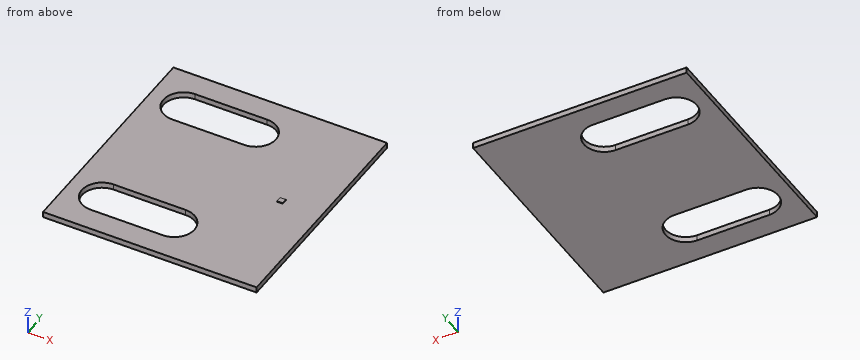
from build123d import *

# Parameters (mm, degrees)
SKETCH1_W           = 37
SKETCH1_H           = 40
BOSS_EXTRUDE1_DEPTH = 1
SKETCH2_W           = 1
SKETCH2_H           = 1
BOSS_EXTRUDE2_DEPTH = 0.1
CUT_EXTRUDE1_DEPTH  = 2


with BuildPart() as part:
    # Sketch1 → Boss-Extrude1 (new body)
    with BuildSketch(Plane.XY):
        with Locations((-11.5, 0)):
            Rectangle(SKETCH1_W, SKETCH1_H)
    extrude(amount=BOSS_EXTRUDE1_DEPTH)

    # Sketch2 → Boss-Extrude2 (add)
    with BuildSketch(Plane.XY.offset(1)):
        Rectangle(SKETCH2_W, SKETCH2_H)
    extrude(amount=BOSS_EXTRUDE2_DEPTH)

    # Sketch3 → Cut-Extrude1 (cut, through all)
    with BuildSketch(Plane.XY.offset(1)):
        with BuildLine():
            Line((-24, 16), (-11.5, 16))
            ThreePointArc((-11.5, 16), (-8, 12.5), (-11.5, 9))
            Line((-11.5, 9), (-24, 9))
            ThreePointArc((-24, 9), (-27.5, 12.5), (-24, 16))
        make_face()
    cut_extrude1 = extrude(amount=-CUT_EXTRUDE1_DEPTH, mode=Mode.SUBTRACT)

    # Mirror1: Cut-Extrude1 across plane
    add(cut_extrude1.mirror(Plane.ZX), mode=Mode.SUBTRACT)


solid = part.part
Read the model definition and answer for the solid it produces. Units are mm, in the model's axes. Round coordinates to 2 decimals unless told otherwise and drop trailing zeros. Loops run counter-clockwise (first coordinate to the right, second up) from the corner with the lowest first, then second, coordinate; pieces in that order, holes last.
Q1. Section A-A on y = 12.5 is taken. Write down the section's boundary in (x, z), and give its area (3 significant figures).
Q2. Section B-B on x = -17 is taken. Write down the section's boundary in (y, z).
Q3. Section D-D on x = -9.5 is taken. Write down the section's boundary in (y, z), and give its area (3 significant figures).
Q4. This flat-tipped pin is pushed along its axis until it touches: pin 1 (8 mm diameter, centred on x = -6, y = 7, fed in from +Z). Where does it stop, or does it pass through?
Q5. Consider probe 1 along Y at (x, z) = (-20.5, 0.5); probe 2 along Z at (x, y) = (-26, 6); probe 3 along X at (y, z) = (13, 0.7). Determine where each line is inside the solid, lowest interval first.
Q6. Section C-C on z = 0.25 is taken. Write down the section's boundary in (x, y).
Output:
1. outline: (-30, 0) - (-27.5, 0) - (-27.5, 1) - (-30, 1) - close; (-8, 0) - (7, 0) - (7, 1) - (-8, 1) - close
1. area: 17.5 mm2
2. outline: (-20, 0) - (-16, 0) - (-16, 1) - (-20, 1) - close; (-9, 0) - (9, 0) - (9, 1) - (-9, 1) - close; (16, 0) - (20, 0) - (20, 1) - (16, 1) - close
3. outline: (-20, 0) - (-15.37, 0) - (-15.37, 1) - (-20, 1) - close; (-9.63, 0) - (9.63, 0) - (9.63, 1) - (-9.63, 1) - close; (15.37, 0) - (20, 0) - (20, 1) - (15.37, 1) - close
3. area: 28.5 mm2
4. pin 1: stops at z = 1
5. probe 1: y = -20 to -16, -9 to 9, 16 to 20
5. probe 2: z = 0 to 1
5. probe 3: x = -30 to -27.46, -8.04 to 7
6. outline: (-30, -20) - (7, -20) - (7, 20) - (-30, 20) - close; hole (-24, -16) - (-11.5, -16) arc R3.5 ccw to (-11.5, -9) - (-24, -9) arc R3.5 ccw to start; hole (-24, 9) - (-11.5, 9) arc R3.5 ccw to (-11.5, 16) - (-24, 16) arc R3.5 ccw to start
